from build123d import *

# Parameters (mm, degrees)
F0_W     = 14
F0_H     = 3
F0_W_2   = 3
F1_DEPTH = 20
F2_DEPTH = 3
F3_W     = 3
F3_H     = 3
F4_DEPTH = 100
F5_W     = 3
F5_H     = 3.5
F6_DEPTH = 100
F7_R     = 1.5
F9_DEPTH = 1


with BuildPart() as f1:
    # F0 (on Front) → F1 (new body)
    with BuildSketch(Plane.XZ):
        Polygon((10, 1.5), (10, 4.5), (-10, 4.5), (-10, 1.5), (-7, 1.5), (7, 1.5), align=None)
        Rectangle(F0_W, F0_H)
        with Locations((11.5, 0)):
            Rectangle(F0_W_2, F0_H)
        with Locations((8.5, 0)):
            Rectangle(F0_W_2, F0_H)
        with Locations((-8.5, 0)):
            Rectangle(F0_W_2, F0_H)
        Polygon((10, -4.5), (10, -1.5), (7, -1.5), (-7, -1.5), (-10, -1.5), (-10, -4.5), align=None)
    extrude(amount=-F1_DEPTH)

    # F0 (on Front) → F2 (join)
    with BuildSketch(Plane.XZ):
        with Locations((-8.5, 0)):
            Rectangle(F0_W_2, F0_H)
        Rectangle(F0_W, F0_H)
        with Locations((8.5, 0)):
            Rectangle(F0_W_2, F0_H)
        with Locations((11.5, 0)):
            Rectangle(F0_W_2, F0_H)
    extrude(amount=F2_DEPTH)

    # F3 (on face) → F4 (cut)
    with BuildSketch(Plane.YZ.offset(13)):
        Polygon((23, -1.75), (23, 1.75), (17, 1.75), (17, 1.5), (20, 1.5), (20, -1.5), (17, -1.5), (17, -1.75), align=None)
        with Locations((18.5, 0)):
            Rectangle(F3_W, F3_H)
    extrude(amount=-F4_DEPTH, mode=Mode.SUBTRACT)

    # F5 (on face) → F6 (cut)
    with BuildSketch(Plane(origin=(0, 17, 0), x_dir=(-1, 0, 0), z_dir=(0, 1, 0))):
        with Locations((11.5, 0)):
            Rectangle(F5_W, F5_H)
        with Locations((8.5, 0)):
            Rectangle(F5_W, F5_H)
    extrude(amount=-F6_DEPTH, mode=Mode.SUBTRACT)

    # F7
    f7_edges = [f1.edges().sort_by_distance(p)[0] for p in [
        (-7, -3, 0),
        (13, -3, 0),
        (10, 0, 3),
        (10, 0, -3),
        (-10, 0, -3.125),
        (-10, 0, 3.125),
        (-7, 17, 0),
        (-10, 20, 3.125),
        (-10, 20, -3.125),
        (13, 17, 0),
        (10, 20, 3.125),
        (10, 20, -3.125),
    ]]
    fillet(f7_edges, radius=F7_R)

    # F8 (on face) → F9 (cut)
    with BuildSketch(Plane.XY.offset(4.5)):
        with BuildLine():
            Line((-1.4625191229, 3), (2.9206384037, 3))
            add(Edge.make_bspline(
                [(5.3432423682, 3.5985243056), (4.0594142819, 3.1793151345), (2.9206384037, 3)],
                knots=[0, 0, 0, 0.958192391, 0.958192391, 0.958192391], degree=2))
            Line((5.3432423682, 3.5985243056), (5.3432423682, 10.7960069444))
            Line((5.3432423682, 10.7960069444), (-0.1650041596, 10.7960069444))
            Line((-0.1650041596, 10.7960069444), (-0.1650041596, 8.3441840278))
            Line((-0.1650041596, 8.3441840278), (2.4660722293, 8.3441840278))
            Line((2.4660722293, 8.3441840278), (2.4660722293, 5.4487847222))
            add(Edge.make_bspline(
                [(0.5945444515, 5.2604166667), (1.5181555626, 5.2604166667), (2.4660722293, 5.4487847222)],
                knots=[0, 0, 0, 1, 1, 1], degree=2))
            add(Edge.make_bspline(
                [(-2.095776729, 6.4513888889), (-1.1706465207, 5.2604166667), (0.5945444515, 5.2604166667)],
                knots=[0, 0, 0, 1, 1, 1], degree=2))
            add(Edge.make_bspline(
                [(-3.0209069374, 9.9027777778), (-3.0209069374, 7.6423611111), (-2.095776729, 6.4513888889)],
                knots=[0, 0, 0, 1, 1, 1], degree=2))
            add(Edge.make_bspline(
                [(-1.8724694374, 13.3480902778), (-3.0209069374, 12.0659722222), (-3.0209069374, 9.9027777778)],
                knots=[0, 0, 0, 1, 1, 1], degree=2))
            add(Edge.make_bspline(
                [(1.1839541737, 14.6302083333), (-0.7240319374, 14.6302083333), (-1.8724694374, 13.3480902778)],
                knots=[0, 0, 0, 1, 1, 1], degree=2))
            add(Edge.make_bspline(
                [(4.3467145904, 13.8706597222), (2.8276173682, 14.6302083333), (1.1839541737, 14.6302083333)],
                knots=[0, 0, 0, 1, 1, 1], degree=2))
            Line((4.3467145904, 13.8706597222), (5.3250132015, 16.2252604167))
            add(Edge.make_bspline(
                [(1.2021833404, 17.0789930556), (3.3410722293, 17.0789930556), (5.3250132015, 16.2252604167)],
                knots=[0, 0, 0, 1, 1, 1], degree=2))
            add(Edge.make_bspline(
                [(-4.1268097151, 15.1998697917), (-2.2036326318, 17.0789930556), (1.2021833404, 17.0789930556)],
                knots=[0, 0, 0, 1, 1, 1], degree=2))
            add(Edge.make_bspline(
                [(-6.0499867985, 9.9605034722), (-6.0499867985, 13.3207465278), (-4.1268097151, 15.1998697917)],
                knots=[0, 0, 0, 1, 1, 1], degree=2))
            add(Edge.make_bspline(
                [(-4.392651729, 4.6558159722), (-6.0499867985, 6.5030381944), (-6.0499867985, 9.9605034722)],
                knots=[0, 0, 0, 1, 1, 1], degree=2))
            add(Edge.make_bspline(
                [(-1.4625191229, 3), (-3.2688097577, 3.4032111719), (-4.392651729, 4.6558159722)],
                knots=[0.3218981532, 0.3218981532, 0.3218981532, 1, 1, 1], degree=2))
        make_face()
    extrude(amount=-F9_DEPTH, mode=Mode.SUBTRACT)


solid = f1.part
Geometry check sheet. Reference: the model listing, model coordinates, mm. A direction names the side the tool comes from. Give positions to 0.01 mm unless a question says otherwise; leave off trailing zeros. Loops run counter-clockwise (first coordinate to the right, second up) from the corner with the lowest first, then second, coordinate; pieces in that order, holes last. Notation, with made-up numbers: (30, 65) -> (81, 65) arc R20 cw to (81, 99) -> close; hole circle Ø5 at (82.5, -14). An arc over 180 degrees is marked (long way). Answer in a Markdown table with one row per item. Add a question column.
1) Set-up check for faces 1 (the face through (9.55, 0.43, 3.02)), 2 (the face through (9.57, 0.45, -2.98)), 3 (the face through (-0.165, 10, 4)): record each of +Z, -Z, +X, -X, +Y, -Y from which the full face is reachable in a straight line by a thin tool's end or side.
2) Cross-section at B-B on z = -0.75. Record the boundary of the cut face in (x, y).
3) Draft check along Z on faces 4 (the face through (0, 10, -4.5)), 5 (the face through (10, 10, -3)), 6 (the face through (-6.55, 16.57, 0.02)), 7 (the face through (6.8, -0.4, 1.5)). Enter one of: pulls with the +Z half, pulls with the -Z half, needs draft (parallel to the pull), parting line crosses it, or undercut.
4) Cross-section at A-A on x = -7.75. Record the boundary of the cut face in (y, z), and give its area (3 significant figures).
5) Cross-section at C-C on x = 6.75. Record the boundary of the cut face in (y, z), and give its area (4 significant figures).
6) Gauge pin test, flat ends, axial feed: P1, Ø0.5, axis at x = 3.5, z = 4, coming from the -Y side; P2, Ø0.9, axis at y = 11, z = -3.5, coming from the +X side. Record the tip position at first contact, or that the pin passes through.
7) Material ranges on probe 1 along Z at (x, y) = (7.25, 18.5); probe 2 along Z at (x, y) = (2.5, 10); probe 3 along Z at (x, y) = (10.5, 4), recorded low to high. Write a range as from..to.
8) Cross-section at D-D on y = -1. Record the boundary of the cut face in (x, z), and give its area (3 significant figures).
Outcome:
| question | item | result |
|---|---|---|
| 1 | face 1 | +Z, +X, -Y |
| 1 | face 2 | -Z, +X, -Y |
| 1 | face 3 | +Z |
| 2 | outline | (-7, -1.5) arc R1.5 ccw to (-5.5, -3) -> (11.5, -3) arc R1.5 ccw to (13, -1.5) -> (13, 15.5) arc R1.5 ccw to (11.5, 17) -> (-5.5, 17) arc R1.5 ccw to (-7, 15.5) -> close |
| 3 | face 4 | pulls with the -Z half |
| 3 | face 5 | needs draft |
| 3 | face 6 | undercut |
| 3 | face 7 | pulls with the +Z half |
| 4 | outline | (0, -4.5) -> (20, -4.5) -> (20, -1.75) -> (0, -1.75) -> close; (0, 1.75) -> (20, 1.75) -> (20, 4.5) -> (0, 4.5) -> close |
| 4 | area | 110 mm^2 |
| 5 | outline | (-3, -1.5) -> (0, -1.5) -> (0, -4.5) -> (20, -4.5) -> (20, -1.75) -> (17, -1.75) -> (17, 1.75) -> (20, 1.75) -> (20, 4.5) -> (0, 4.5) -> (0, 1.5) -> (-3, 1.5) -> close |
| 5 | area | 178.5 mm^2 |
| 6 | P1 | stops at y = 0 |
| 6 | P2 | stops at x = 10 |
| 7 | probe 1 | z = -4.5..-1.75, 1.75..4.5 |
| 7 | probe 2 | z = -4.5..3.5 |
| 7 | probe 3 | z = -1.5..1.5 |
| 8 | outline | (-7, -1.5) -> (13, -1.5) -> (13, 1.5) -> (-7, 1.5) -> close |
| 8 | area | 60.0 mm^2 |
